CAD build for the part. Positions are in the model's coordinates, mm. A direction names the side the tool comes from. Round coordinates to 2 decimals unless told otherwise and drop trailing zeros. Loops run counter-clockwise (first coordinate to the right, second up) from the corner with the lowest first, then second, coordinate; pieces in that order, holes last. Notation, with made-up numbers: M 77.25,-17 L 118.25,-17 A8 cw 118.25,-6 Z; hole C -38.75,64.5 d7. An arc over 180 degrees is marked long. Use one line per item in the form item = value.
from build123d import *

# Parameters (mm, degrees)
SKETCH1_W           = 67
SKETCH1_H           = 67
SKETCH1_W_2         = 3
SKETCH1_H_2         = 10
SKETCH1_W_3         = 10
SKETCH1_H_3         = 3
BOSS_EXTRUDE1_DEPTH = 3
SKETCH3_W           = 6.460545278
SKETCH3_H           = 1.169767542
SKETCH3_W_2         = 7.74987154
SKETCH3_H_2         = 4.501562016
SKETCH3_W_3         = 6.14987154
SKETCH3_H_3         = 2.901562016
SKETCH3_R           = 11.812674278
SKETCH3_R_2         = 11.012674278
SKETCH3_R_3         = 8.532957956
SKETCH3_R_4         = 7.732957956
CUT_EXTRUDE1_DEPTH  = 0.3


with BuildPart() as part:
    # Sketch1 → Boss-Extrude1 (new body)
    with BuildSketch(Plane(origin=(0, 0, 0), x_dir=(1, 0, 0), z_dir=(0, 1, 0))):
        Rectangle(SKETCH1_W, SKETCH1_H)
        with Locations((-35, -21.5)):
            Rectangle(SKETCH1_W_2, SKETCH1_H_2)
        with Locations((-35, -1.5)):
            Rectangle(SKETCH1_W_2, SKETCH1_H_2)
        with Locations((-35, 18.5)):
            Rectangle(SKETCH1_W_2, SKETCH1_H_2)
        with Locations((-18.5, -35)):
            Rectangle(SKETCH1_W_3, SKETCH1_H_3)
        with Locations((1.5, -35)):
            Rectangle(SKETCH1_W_3, SKETCH1_H_3)
        with Locations((21.5, -35)):
            Rectangle(SKETCH1_W_3, SKETCH1_H_3)
        with Locations((35, -18.5)):
            Rectangle(SKETCH1_W_2, SKETCH1_H_2)
        with Locations((35, 1.5)):
            Rectangle(SKETCH1_W_2, SKETCH1_H_2)
        with Locations((35, 21.5)):
            Rectangle(SKETCH1_W_2, SKETCH1_H_2)
        with Locations((18.5, 35)):
            Rectangle(SKETCH1_W_3, SKETCH1_H_3)
        with Locations((-1.5, 35)):
            Rectangle(SKETCH1_W_3, SKETCH1_H_3)
        with Locations((-21.5, 35)):
            Rectangle(SKETCH1_W_3, SKETCH1_H_3)
    extrude(amount=BOSS_EXTRUDE1_DEPTH)

    # Sketch3 → Cut-Extrude1 (cut)
    # profile 1 of 5: a face of its own
    with BuildSketch(Plane.XZ):
        with BuildLine():
            Line((17.951474003, -11.996306148), (19.468912415, -11.996306148))
            ThreePointArc((19.468912415, -11.996306148), (21.873075471, -11.000469204), (22.868912415, -8.596306148))
            Line((22.868912415, -8.596306148), (22.868912415, 12.012813943))
            ThreePointArc((22.868912415, 12.012813943), (21.873075471, 14.416976999), (19.468912415, 15.412813943))
            Line((19.468912415, 15.412813943), (-19.75568403, 15.412813943))
            ThreePointArc((-19.75568403, 15.412813943), (-22.159847086, 14.416976999), (-23.15568403, 12.012813943))
            Line((-23.15568403, 12.012813943), (-23.15568403, -8.596306148))
            ThreePointArc((-23.15568403, -8.596306148), (-22.159847086, -11.000469204), (-19.75568403, -11.996306148))
            Line((-19.75568403, -11.996306148), (-7.131170101, -11.996306148))
            Line((-7.131170101, -11.996306148), (-6.58045367, -15.77368629))
            ThreePointArc((-6.58045367, -15.77368629), (-5.775436093, -17.242792), (-4.205560916, -17.827443017))
            Line((-4.205560916, -17.827443017), (4.072492002, -17.827443017))
            ThreePointArc((4.072492002, -17.827443017), (5.634337803, -17.249704715), (6.444235152, -15.794641095))
            Line((6.444235152, -15.794641095), (7.032301062, -11.996306148))
            Line((7.032301062, -11.996306148), (9.890928725, -11.996306148))
            Line((9.890928725, -11.996306148), (9.890928725, -13.96607369))
            Line((9.890928725, -13.96607369), (17.951474003, -13.96607369))
            Line((17.951474003, -13.96607369), (17.951474003, -11.996306148))
        make_face()
        with BuildLine():
            Line((-6.322712542, -11.996306148), (6.222769895, -11.996306148))
            Line((6.222769895, -11.996306148), (5.653654102, -15.672241736))
            ThreePointArc((5.653654102, -15.672241736), (5.113722536, -16.642284149), (4.072492002, -17.027443017))
            Line((4.072492002, -17.027443017), (-4.205560916, -17.027443017))
            ThreePointArc((-4.205560916, -17.027443017), (-5.252144367, -16.637675672), (-5.788822752, -15.658271866))
            Line((-5.788822752, -15.658271866), (-6.322712542, -11.996306148))
        make_face(mode=Mode.SUBTRACT)
        with Locations((13.921201364, -12.581189919)):
            Rectangle(SKETCH3_W, SKETCH3_H, mode=Mode.SUBTRACT)
        with BuildLine():
            ThreePointArc((22.068912415, -8.596306148), (21.307390046, -10.434783779), (19.468912415, -11.196306148))
            Line((19.468912415, -11.196306148), (-19.75568403, -11.196306148))
            ThreePointArc((-19.75568403, -11.196306148), (-21.594161661, -10.434783779), (-22.35568403, -8.596306148))
            Line((-22.35568403, -8.596306148), (-22.35568403, 12.012813943))
            ThreePointArc((-22.35568403, 12.012813943), (-21.594161661, 13.851291574), (-19.75568403, 14.612813943))
            Line((-19.75568403, 14.612813943), (19.468912415, 14.612813943))
            ThreePointArc((19.468912415, 14.612813943), (21.307390046, 13.851291574), (22.068912415, 12.012813943))
            Line((22.068912415, 12.012813943), (22.068912415, -8.596306148))
        make_face(mode=Mode.SUBTRACT)
    # profile 2 of 5: a face of its own
    with BuildSketch(Plane.XZ):
        with BuildLine():
            Line((-3.20545277, -15.827443017), (2.975704553, -15.827443017))
            add(Edge.make_bspline(
                [(2.953511817, -12.870475248), (3.156880299, -12.869857322), (3.585089851, -12.956102965), (4.018056229, -13.335311226), (4.232845726, -13.825946117), (4.282993557, -14.510967663), (4.056789396, -15.180852207), (3.536001149, -15.684997342), (3.16114062, -15.80680282), (2.975704553, -15.827443017)],
                knots=[0.000309469, 0.000309469, 0.000309469, 0.000309469, 0.126123229, 0.251936989, 0.37775075, 0.50356451, 0.75519203, 0.881005791, 1.006819551, 1.006819551, 1.006819551, 1.006819551], degree=3))
            Line((2.953511817, -12.870475248), (-3.208812782, -12.870477681))
            add(Edge.make_bspline(
                [(-3.20545277, -15.827443017), (-3.402440677, -15.796950089), (-3.804790668, -15.67436393), (-4.360046403, -15.161364486), (-4.548558911, -14.293381235), (-4.249990898, -13.494614941), (-3.796080691, -13.08166476), (-3.514079359, -12.94650227), (-3.330583264, -12.891839413), (-3.250572572, -12.877657517), (-3.208812782, -12.870477681)],
                knots=[-0.01081197, -0.01081197, -0.01081197, -0.01081197, 0.116511645, 0.24383526, 0.49848249, 0.75312972, 0.880453335, 0.944115143, 0.975946047, 1.00777695, 1.00777695, 1.00777695, 1.00777695], degree=3))
        make_face()
        with BuildLine():
            add(Edge.make_bspline(
                [(2.954312548, -13.670477681), (3.002162708, -13.670286106), (3.107702292, -13.680346372), (3.235248962, -13.726706918), (3.341954697, -13.812630756), (3.434286544, -13.998064842), (3.47500749, -14.35295522), (3.304919264, -14.84862877), (3.068019803, -15.006185035), (2.927947638, -15.027443017)],
                knots=[-0.000203812, -0.000203812, -0.000203812, -0.000203812, 0.061637445, 0.123478703, 0.247161218, 0.370843733, 0.494526248, 0.741891278, 0.989256308, 0.989256308, 0.989256308, 0.989256308], degree=3))
            Line((2.927947638, -15.027443017), (-3.141370514, -15.027443017))
            add(Edge.make_bspline(
                [(-3.141370514, -15.027443017), (-3.191002063, -15.018349114), (-3.295796079, -14.989541193), (-3.43833154, -14.916637531), (-3.558968521, -14.800275144), (-3.643853224, -14.612459797), (-3.674059975, -14.29626228), (-3.520794101, -13.870784083), (-3.275666554, -13.702096641), (-3.135980342, -13.670477681)],
                knots=[0.01613903, 0.01613903, 0.01613903, 0.01613903, 0.077002925, 0.137866819, 0.259594608, 0.381322398, 0.503050187, 0.746505765, 0.989961344, 0.989961344, 0.989961344, 0.989961344], degree=3))
            Line((-3.135980342, -13.670477681), (2.954312548, -13.670477681))
        make_face(mode=Mode.SUBTRACT)
    # profile 3 of 5: a face of its own
    with BuildSketch(Plane.XZ):
        with Locations((-16.962226762, -3.831057055)):
            Rectangle(SKETCH3_W_2, SKETCH3_H_2)
        with Locations((-16.962226762, -3.831057055)):
            Rectangle(SKETCH3_W_3, SKETCH3_H_3, mode=Mode.SUBTRACT)
    # profile 4 of 5: a face of its own
    with BuildSketch(Plane.XZ):
        with Locations(Location((-0.032284279, 1.802644777, 0), (0, 0, 270))):
            Circle(SKETCH3_R)
        with Locations(Location((-0.032284279, 1.802644777, 0), (0, 0, 270))):
            Circle(SKETCH3_R_2, mode=Mode.SUBTRACT)
    # profile 5 of 5: a face of its own
    with BuildSketch(Plane.XZ):
        with Locations(Location((-0.153217329, 1.801981193, 0), (0, 0, 270))):
            Circle(SKETCH3_R_3)
        with Locations(Location((-0.153217329, 1.801981193, 0), (0, 0, 270))):
            Circle(SKETCH3_R_4, mode=Mode.SUBTRACT)
    extrude(amount=-CUT_EXTRUDE1_DEPTH, mode=Mode.SUBTRACT)


solid = part.part
1. Pull direction Z, two halves, no side cores. Call faces 5 (the face through (-35, 1, -23.5)), 6 (the face through (-35, 1, -3.5)), 7 (the face through (-36.5, 1, 2)), 8 (the face through (21, 1, 36.5)): +Z half, -Z half, draft (parallel to the pull), parting line (faces both ways), or undercut.
Completed:
face_5 = -Z half
face_6 = undercut
face_7 = draft
face_8 = +Z half
2. Cut at A-A on z = -29. Write the cut outline in (x, y), and give its area (3 significant figures).
Completed:
outline = M -33.5,0 L 33.5,0 L 33.5,3 L -33.5,3 Z
area = 201 mm2
3. Probe line 1 along Z through (x, y) = (26, 1.8); line 2 along X through (y, z) = (0.45, -32). List the from-to ranges inside material, lowest first. Write a range as from..to.
Completed:
line_1 = -33.5..36.5
line_2 = -33.5..33.5
4. Drop a flat-ended pin along its axis: P1, Ø1, axis at x = 4.5, y = 2.5, coming from the -Z side. Give the stop position or say it passes through.
Completed:
P1 = -33.5
5. Cut at B-B on z = 5.5. Write the cut outline in (x, y).
Completed:
outline = M -36.5,0 L -23.16,0 L -23.16,0.3 L -22.36,0.3 L -22.36,0 L -11.25,0 L -11.25,0.3 L -10.41,0.3 L -10.41,0 L -7.84,0 L -7.84,0.3 L -6.94,0.3 L -6.94,0 L 6.64,0 L 6.64,0.3 L 7.54,0.3 L 7.54,0 L 10.34,0 L 10.34,0.3 L 11.19,0.3 L 11.19,0 L 22.07,0 L 22.07,0.3 L 22.87,0.3 L 22.87,0 L 33.5,0 L 33.5,3 L -36.5,3 Z
6. Tool access for faces 1 (the face through (-16.5, 1, -35)), 2 (the face through (-35, 1, 16.5)), 3 (the face through (33.5, 1, 9)), 4 (the face through (-23.5, 1, 35)): list every direction of +Z, -Z, +X, -X, +Y, -Y with a clear straight run to the whole face (end or side of a thin tool).
Completed:
face_1 = -Z, +Y, -Y
face_2 = -X, +Y, -Y
face_3 = +X, +Y, -Y
face_4 = +Z, -X, +Y, -Y
